```python
from build123d import *

# Parameters (mm, degrees)
F0_W     = 400
F0_H     = 150
F1_DEPTH = 400
F2_W     = 100
F2_H     = 50
F3_DEPTH = 100
F4_W     = 100
F4_H     = 50
F5_DEPTH = 100
F6_R     = 25
F7_DEPTH = 400.001
F8_R     = 25
F9_DEPTH = 400.001
F10_SIZE = 5


with BuildPart() as f1:
    # F0 (on Front) → F1 (new body)
    with BuildSketch(Plane.XZ):
        Rectangle(F0_W, F0_H)
    extrude(amount=F1_DEPTH)

    # F2 (on face) → F3 (cut)
    with BuildSketch(Plane.XZ.offset(400)):
        with Locations((150, 0)):
            Rectangle(F2_W, F2_H)
        with Locations((-150, 0)):
            Rectangle(F2_W, F2_H)
    extrude(amount=-F3_DEPTH, mode=Mode.SUBTRACT)

    # F4 (on face) → F5 (cut)
    with BuildSketch(Plane(origin=(0, 0, 0), x_dir=(-1, 0, 0), z_dir=(0, 1, 0))):
        with Locations((150, 0)):
            Rectangle(F4_W, F4_H)
        with Locations((-150, 0)):
            Rectangle(F4_W, F4_H)
    extrude(amount=-F5_DEPTH, mode=Mode.SUBTRACT)

    # F6 (on face) → F7 (cut, through all)
    with BuildSketch(Plane(origin=(0, 0, 0), x_dir=(-1, 0, 0), z_dir=(0, 1, 0))):
        Circle(F6_R)
    extrude(amount=-F7_DEPTH, mode=Mode.SUBTRACT)

    # F8 (on face) → F9 (cut, through all)
    with BuildSketch(Plane(origin=(-200, 0, 0), x_dir=(0, -1, 0), z_dir=(-1, 0, 0))):
        with Locations((200, 0)):
            Circle(F8_R)
    extrude(amount=-F9_DEPTH, mode=Mode.SUBTRACT)

    # F10
    f10_edges = [f1.edges().sort_by_distance(p)[0] for p in [
        (-200, -200, 75),
        (-200, -200, -75),
        (0, 0, 75),
        (0, 0, -75),
        (-200, -175, 0),
        (25, 0, 0),
        (200, -200, -75),
        (200, -200, 75),
        (200, -175, 0),
        (0, -400, -75),
        (0, -400, 75),
        (25, -400, 0),
    ]]
    chamfer(f10_edges, length=F10_SIZE)


solid = f1.part
```
Input: part model. Units: mm. Frame: model coordinates. A direction names the side the tool comes from. Coordinates: 2 decimals unless noted, no trailing zeros. Loops run counter-clockwise (first coordinate to the right, second up) from the corner with the lowest first, then second, coordinate; pieces in that order, holes last. Notation, with made-up numbers: M -37,83 L 9,83 A22 ccw 9,93 Z; hole C 20.5,46 d11. An arc over 180 degrees is marked long. Answer in a Markdown table with one row per item.
1. Draft query along X for faces 4 (the flat face through (151, -49, -25)), 5 (the conical face through (3.286, -4.757, 25.028)), 6 (the flat face through (-100, -351, 0)). Return one class per face: pulls with the +X half, pulls with the -X half, needs draft (parallel to the pull), parting line crosses it, or undercut.
Response:
| item | result |
|---|---|
| face 4 | needs draft |
| face 5 | undercut |
| face 6 | pulls with the -X half |
2. Section C-C, the plane z = 0. Count the separate pieces of the cut face and the enclosed holes in it, then the cut area to 3 significant figures.
Response:
| item | result |
|---|---|
| separate pieces | 4 |
| enclosed holes | 0 |
| area | 82,400 mm2 |
3. Material intervals for line 1 (X direction, y = -322, z = 0); line 2 (Z direction, x = -135.5, y = -355.5); line 3 (Y direction, x = -134, z = 0), sorted ascending.
Response:
| item | result |
|---|---|
| line 1 | x = -100 to -25, 25 to 100 |
| line 2 | z = -75 to -25, 25 to 75 |
| line 3 | y = -300 to -225, -175 to -100 |
4. Reachability of faces 1 (the flat face through (-151, -351, 25)), 2 (the flat face through (149, -351, 25)), 3 (the flat face through (-149, -49, -25)) from +Z, -Z, +X, -X, +Y, -Y: full face, straight path, thin tool, end or side. Return the list, or none.
Response:
| item | result |
|---|---|
| face 1 | -X, -Y |
| face 2 | +X, -Y |
| face 3 | -X, +Y |
5. Section B-B, the plane y = -55. Output: boundary loops of the cut face in (x, z), then the cut area to 3 significant figures.
Response:
| item | result |
|---|---|
| outline | M -200,-70 L -195,-75 L 195,-75 L 200,-70 L 200,-25 L 100,-25 L 100,25 L 200,25 L 200,70 L 195,75 L -195,75 L -200,70 L -200,25 L -100,25 L -100,-25 L -200,-25 Z; hole C 0,0 d50 |
| area | 48,000 mm2 |
6. First-contact query: pin 1 (25 mm diameter, centred on x = -143.5, z = -6.5, fed in from -Y); pin 2 (3 mm diameter, centred on y = -78.5, z = -14, fed in from -X); pin 3 (15 mm diameter, centred on x = 145, z = 0.5, fed in from +Y). Flat tips, straight axial feed; report the tip coordinate or a pass-through.
Response:
| item | result |
|---|---|
| pin 1 | stops at y = -300 |
| pin 2 | stops at x = -100 |
| pin 3 | stops at y = -100 |
7. Section D-D, the plane y = -278. Output: boundary loops of the cut face in (x, z).
Response:
| item | result |
|---|---|
| outline | M -200,-70 L -195,-75 L 195,-75 L 200,-70 L 200,70 L 195,75 L -195,75 L -200,70 Z; hole C 0,0 d50 |
8. Section A-A, the plane x = -148.5. Output: boundary loops of the cut face in (y, z).
Response:
| item | result |
|---|---|
| outline | M -400,-70 L -395,-75 L -5,-75 L 0,-70 L 0,-25 L -100,-25 L -100,25 L 0,25 L 0,70 L -5,75 L -395,75 L -400,70 L -400,25 L -300,25 L -300,-25 L -400,-25 Z; hole C -200,0 d50 |
